Work out the finished part from the listing and answer in its coordinate system (mm). Give positions to 0.01 mm unless a question says otherwise; leave off trailing zeros. Write each loop counter-clockwise with the first axis right and the second up, starting at its lowest first coordinate (ties: lowest second). Pieces come first, ordered by that corner, then holes.
1) Given pin 1 Ø1.9 at (x, y) = (82.5, -1.5) entering from +Z; pin 2 Ø1.1 at (y, z) = (-2.5, -27) entering from -X; pin 3 Ø1.1 at (x, y) = (83.5, -2.5) entering from -Z, each flat-ended and moving along its own axis, determine where each tip first touches the part or whether it passes through.
2) Find section A-A (x = -28). Determine the outline of the cut face in (y, z).
3) A straight line is drawn through the part: probe 1 along Z at (x, y) = (59.5, -2.4). Find the intervals that lie inside material, in ascending order.
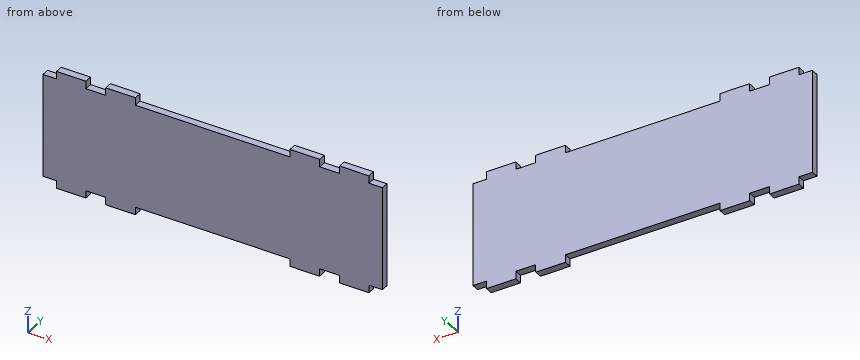
```python
from build123d import *

# Parameters (mm, degrees)
F0_W     = 14.8
F0_H     = 3.81
F0_W_2   = 15
F1_DEPTH = 3.81


# Not quite as in the source:
# - a feature names something its author has since deleted; it is built from what else it names


with BuildPart() as f1:
    # F0 (on Front) → F1 (new body)
    with BuildSketch(Plane.XZ):
        Polygon((85.62, 0), (85.62, 26), (78.8, 26), (64, 26), (54, 26), (39, 26), (0, 26), (0, 0), align=None)
        Polygon((-85.62, 0), (0, 0), (0, 26), (-39, 26), (-54, 26), (-64, 26), (-78.8, 26), (-85.62, 26), align=None)
        Polygon((0, -26), (0, 0), (-85.62, 0), (-85.62, -26), (-78.8, -26), (-64, -26), (-54, -26), (-39, -26), align=None)
        Polygon((85.62, -26), (85.62, 0), (0, 0), (0, -26), (39, -26), (54, -26), (64, -26), (78.8, -26), align=None)
        with Locations((71.4, 27.905)):
            Rectangle(F0_W, F0_H)
        with Locations((-71.4, -27.905)):
            Rectangle(F0_W, F0_H)
        with Locations((-71.4, 27.905)):
            Rectangle(F0_W, F0_H)
        with Locations((71.4, -27.905)):
            Rectangle(F0_W, F0_H)
        with Locations((-46.5, 27.905)):
            Rectangle(F0_W_2, F0_H)
        with Locations((-46.5, -27.905)):
            Rectangle(F0_W_2, F0_H)
        with Locations((46.5, -27.905)):
            Rectangle(F0_W_2, F0_H)
        with Locations((46.5, 27.905)):
            Rectangle(F0_W_2, F0_H)
    extrude(amount=F1_DEPTH)


solid = f1.part
```
Results:
1. pin 1: stops at z = 26
1. pin 2: stops at x = -78.8
1. pin 3: stops at z = -26
2. outline: (-3.81, -26) - (0, -26) - (0, 26) - (-3.81, 26) - close
3. probe 1: z = -26 to 26
